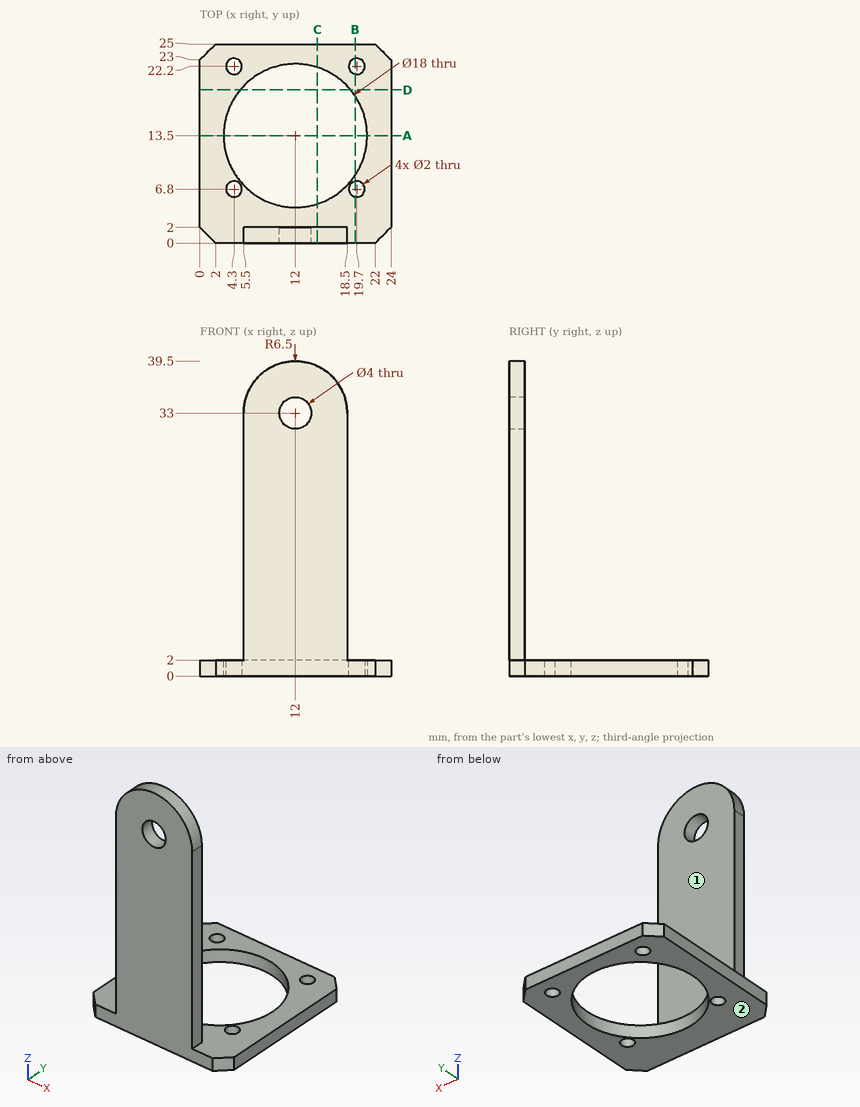
Design review of the part shown in the three views and the two pictorial views. Dimensions are in mm from the part's minimum x, y and z. A direction names the side the tool comes from. Coordinates: 2 decimals unless noted, no trailing zeros. Loops run counter-clockwise (first coordinate to the right, second up) from the corner with the lowest first, then second, coordinate; pieces in that order, holes last.
Q1. To check wall thickness, follow line 1 (Y direction, x = 12, z = 1.2); line 2 (Y direction, x = 4.3, z = 1.35); line 3 (Z direction, x = 16.75, y = 23.75). State the ranges of each line that lie inside material, in increasing order.
Reported:
line 1: y = 0 to 4.5, 22.5 to 25
line 2: y = 0 to 5.8, 7.8 to 8.84, 18.16 to 21.2, 23.2 to 25
line 3: z = 0 to 2
Q2. We need section A-A on y = 13.5. State the section outline as (x, z) points, and give its area (3 significant figures).
Reported:
outline: (0, 0) - (3, 0) - (3, 2) - (0, 2) - close; (21, 0) - (24, 0) - (24, 2) - (21, 2) - close
area: 12.0 mm2
Q3. We need section B-B on x = 19.5. State the section outline as (y, z) points, and give its area (3 significant figures).
Reported:
outline: (0, 0) - (5.82, 0) - (5.82, 2) - (0, 2) - close; (7.78, 0) - (8.53, 0) - (8.53, 2) - (7.78, 2) - close; (18.47, 0) - (21.22, 0) - (21.22, 2) - (18.47, 2) - close; (23.18, 0) - (25, 0) - (25, 2) - (23.18, 2) - close
area: 22.3 mm2
Q4. For pin 1 (1.6 mm diameter, centred on x = 4.3, y = 22.2, fed in from +Z); pin 2 (1.6 mm diameter, centred on y = 0.5, z = 22, fed in from +X); pin 3 (1 mm diameter, centred on y = 1, z = 23, fed in from -X); pin 4 (10.5 mm diameter, centred on x = 10, z = 11.5, fed in from +Y), all flat-tipped, find the tip position at first contact; note any pin that passes through.
Reported:
pin 1: passes through
pin 2: stops at x = 18.5
pin 3: stops at x = 5.5
pin 4: stops at y = 2
Q5. Tool access review of the marked faces 1 and 2: name each direction out of +Z, -Z, +X, -X, +Y, -Y from which nothing blocks a thin tool from reaching the whole face with its end or side.
Reported:
face 1: +Z, +X, -X, +Y
face 2: -Z, +X, -X, +Y, -Y
Q6. We need section C-C on x = 14.75. State the section outline as (y, z) points.
Reported:
outline: (0, 0) - (4.93, 0) - (4.93, 2) - (2, 2) - (2, 38.89) - (0, 38.89) - close; (22.07, 0) - (25, 0) - (25, 2) - (22.07, 2) - close
Q7. We need section D-D on y = 19.25. State the section outline as (x, z) points, and give its area (3 significant figures).
Reported:
outline: (0, 0) - (5.08, 0) - (5.08, 2) - (0, 2) - close; (18.92, 0) - (24, 0) - (24, 2) - (18.92, 2) - close
area: 20.3 mm2
